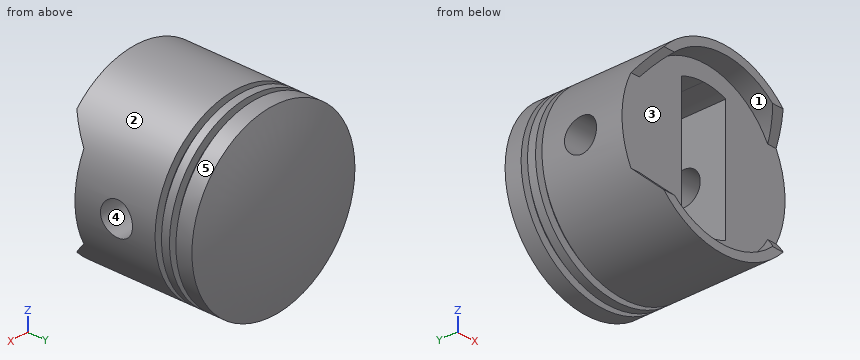
```python
from build123d import *

# Parameters (mm, degrees)
CUT_EXTRUDE_2_DEPTH      = 39.105117767
CUT_EXTRUDE_2_DEPTH_BACK = 39.105117767
SKETCH_4_R               = 4
SKETCH_6_R               = 20
CUT_EXTRUDE_3_DEPTH      = 5
CUT_EXTRUDE_4_DEPTH      = 6
EXTRUDE_1_REACH          = 46.896
EXTRUDE_1_END_RADIUS     = 75


with BuildPart() as part:
    # 草图1 → 旋转3 (revolve)
    with BuildSketch(Plane.XY):
        with BuildLine():
            Line((-22, 9.633147735), (-22, -15.366852265))
            Line((-22, -15.366852265), (0, -15.366852265))
            Line((0, -15.366852265), (0, 22))
            ThreePointArc((0, 22), (-11.113381048, 21.204227615), (-22, 18.833147735))
            Line((-22, 18.833147735), (-22, 14.833147735))
            Line((-22, 14.833147735), (-20, 14.833147735))
            Line((-20, 14.833147735), (-20, 13.233147735))
            Line((-20, 13.233147735), (-22, 13.233147735))
            Line((-22, 13.233147735), (-22, 11.233147735))
            Line((-22, 11.233147735), (-20, 11.233147735))
            Line((-20, 11.233147735), (-20, 9.633147735))
            Line((-20, 9.633147735), (-22, 9.633147735))
        make_face()
    revolve(axis=Axis((0, 22, 0), (0, -1, 0)))

    # 草图4 → 切除-拉伸2 (cut, two sides: drawn at the far end of the back side and taken through both)
    with BuildSketch(Plane(origin=(0, 0, 0), x_dir=(0, 0, -1), z_dir=(1, 0, 0)).offset(-CUT_EXTRUDE_2_DEPTH_BACK)):
        Circle(SKETCH_4_R)
        Polygon((-15, -15.366852265), (-10, -10.366852265), (10, -10.366852265), (15, -15.366852265), align=None)
    extrude(amount=CUT_EXTRUDE_2_DEPTH + CUT_EXTRUDE_2_DEPTH_BACK, mode=Mode.SUBTRACT)

    # 草图6 → 切除-拉伸3 (cut)
    with BuildSketch(Plane.XZ.offset(15.366852265)):
        with Locations(Location((0, 0, 0), (0, 0, 180))):
            Circle(SKETCH_6_R)
    extrude(amount=-CUT_EXTRUDE_3_DEPTH, mode=Mode.SUBTRACT)

    # 草图8 → 切除-拉伸4 (cut, symmetric)
    with BuildSketch(Plane(origin=(0, 0, 0), x_dir=(0, 0, -1), z_dir=(1, 0, 0))):
        with BuildLine():
            Line((-16, 17.273460407), (-16, -10.366852265))
            Line((-16, -10.366852265), (16, -10.366852265))
            Line((16, -10.366852265), (16, 17.273460407))
            ThreePointArc((16, 17.273460407), (0, 19), (-16, 17.273460407))
        make_face()
    extrude(amount=CUT_EXTRUDE_4_DEPTH, both=True, mode=Mode.SUBTRACT)

    # 凸台-拉伸1: up to this cylinder (the profile starts inside it)
    extrude_1_end = Plane(origin=(0, -56, 0), z_dir=(1, 0, 0)) * Cylinder(EXTRUDE_1_END_RADIUS, 253.81433, mode=Mode.PRIVATE)
    # 草图9 → 凸台-拉伸1 (add, up to the surface)
    with BuildSketch(Plane.XZ.offset(10.366852265), mode=Mode.PRIVATE) as extrude_1_sk1:
        with BuildLine():
            Line((6, -16), (6, -14.832396974))
            ThreePointArc((6, -14.832396974), (3.056276215, -15.705386837), (3.1e-08, -16))
            Line((3.1e-08, -16), (6, -16))
        make_face()
    extrude_1_tool1 = extrude(extrude_1_sk1.sketch, amount=-EXTRUDE_1_REACH, mode=Mode.PRIVATE) & extrude_1_end
    add(extrude_1_tool1.solids().sort_by_distance((4.511165, -10.366852, -15.652025))[0])
    # 草图9 → 凸台-拉伸1 (add, up to the surface)
    with BuildSketch(Plane.XZ.offset(10.366852265), mode=Mode.PRIVATE) as extrude_1_sk2:
        with BuildLine():
            Line((-6, -16), (3.1e-08, -16))
            ThreePointArc((3.1e-08, -16), (-3.056276184, -15.705386843), (-6, -14.832396974))
            Line((-6, -14.832396974), (-6, -16))
        make_face()
    extrude_1_tool2 = extrude(extrude_1_sk2.sketch, amount=-EXTRUDE_1_REACH, mode=Mode.PRIVATE) & extrude_1_end
    add(extrude_1_tool2.solids().sort_by_distance((-4.511165, -10.366852, -15.652025))[0])
    # 草图9 → 凸台-拉伸1 (add, up to the surface)
    with BuildSketch(Plane.XZ.offset(10.366852265), mode=Mode.PRIVATE) as extrude_1_sk3:
        with BuildLine():
            ThreePointArc((-6, 14.832396974), (-3.056276199, 15.70538684), (0, 16))
            Line((0, 16), (-6, 16))
            Line((-6, 16), (-6, 14.832396974))
        make_face()
    extrude_1_tool3 = extrude(extrude_1_sk3.sketch, amount=-EXTRUDE_1_REACH, mode=Mode.PRIVATE) & extrude_1_end
    add(extrude_1_tool3.solids().sort_by_distance((-4.511165, -10.366852, 15.652025))[0])
    # 草图9 → 凸台-拉伸1 (add, up to the surface)
    with BuildSketch(Plane.XZ.offset(10.366852265), mode=Mode.PRIVATE) as extrude_1_sk4:
        with BuildLine():
            Line((6, 14.832396974), (6, 16))
            Line((6, 16), (0, 16))
            ThreePointArc((0, 16), (3.056276199, 15.70538684), (6, 14.832396974))
        make_face()
    extrude_1_tool4 = extrude(extrude_1_sk4.sketch, amount=-EXTRUDE_1_REACH, mode=Mode.PRIVATE) & extrude_1_end
    add(extrude_1_tool4.solids().sort_by_distance((4.511165, -10.366852, 15.652025))[0])


solid = part.part
```
Verification items for the finished model (mm, model axes). Face numbers are marked on the shaded views. A direction names the side the tool comes from. Coordinates: 2 decimals unless noted, no trailing zeros. Order: outer loops, then holes, each group sorted by start corner. A loop starts at its lowest first (then second) coordinate and runs counter-clockwise, first axis right, second up. Notation, with made-up numbers: (-26, -25.5) -> (-20, -25.5) arc R30 ccw to (-20, 8.5) -> close; hole circle Ø1 at (85.25, 69). An arc over 180 degrees is marked (long way). Put each result on its own line as item: value. Start each with the question number.
1) Cross-section at B-B (z = 0). State how many separate pieces and enclosed holes the cut face has, plus the area to 3 significant figures.
2) Tool access check on the marked faces 1 and 2. Record the directions out of +Z, -Z, +X, -X, +Y, -Y that give a thin tool (end or side, any length) a straight path to the whole face; none if there is none.
3) Cross-section at C-C (x = 15). Enter the section's corners in (y, z).
4) Go/stop test with flat-tipped pins: pin 1 (6.5 mm diameter, centred on y = 0, z = 0, fed in from +X); pin 2 (9 mm diameter, centred on y = 2, z = -5.5, fed in from -X); pin 3 (3 mm diameter, centred on x = -15, y = 2, fed in from +Z); pin 4 (22 mm diameter, centred on x = 1, z = 2, fed in from -Y). Record where each tip stops, or that it passes through.
5) Cross-section at A-A (y = 16). Enter the section's corners in (x, z).
6) Material ranges on L1, parallel to Y at x = 17.5, z = -8; L2, parallel to X at y = 3.5, z = 11; L3, parallel to Z at x = 11.5, y = 0 (3 decimals), recorded low to high.
7) Cross-section at D-D (y = 0). Enter the section's corners in (x, z), plus the area to 3 significant figures.
8) Release check for a two-part mould opening along X. For the marked faces 3, 4 and 5 record: pulls with the +X half, pulls with the -X half, needs draft (parallel to the pull), parting line crosses it, or undercut.
Geometry check:
1. separate pieces: 3
1. enclosed holes: 0
1. area: 757 mm^2
2. face 1: -Y
2. face 2: +Y, -Y
3. outline: (-15.37, -16.09) -> (9.63, -16.09) -> (9.63, -13.23) -> (11.23, -13.23) -> (11.23, -16.09) -> (13.23, -16.09) -> (13.23, -13.23) -> (14.83, -13.23) -> (14.83, -16.09) -> (18.83, -16.09) arc R76.54 ccw to (18.83, 16.09) -> (14.83, 16.09) -> (14.83, 13.23) -> (13.23, 13.23) -> (13.23, 16.09) -> (11.23, 16.09) -> (11.23, 13.23) -> (9.63, 13.23) -> (9.63, 16.09) -> (-15.37, 16.09) -> (-15.37, 15) -> (-13.6, 13.23) -> (-10.37, 13.23) -> (-10.37, -13.23) -> (-13.6, -13.23) -> (-15.37, -15) -> close; hole circle Ø8 at (0, 0)
4. pin 1: passes through
4. pin 2: stops at x = -21.96
4. pin 3: stops at z = 17.37
4. pin 4: stops at y = -10.37
5. outline: circle Ø44 at (0, 0); hole (-6, -14.83) arc R16 ccw to (6, -14.83) -> (6, 14.83) arc R16 ccw to (-6, 14.83) -> close
6. L1: y = -10.37 to 19.59
6. L2: x = -19.05 to -6, 6 to 19.05
6. L3: z = -18.755 to -4, 4 to 18.755
7. outline: (-21.63, -4) arc R22 ccw to (21.63, -4) -> (6, -4) -> (6, -14.83) arc R16 cw to (-6, -14.83) -> (-6, -4) -> close; (-21.63, 4) -> (-6, 4) -> (-6, 14.83) arc R16 cw to (6, 14.83) -> (6, 4) -> (21.63, 4) arc R22 ccw to start
7. area: 892 mm^2
8. face 3: undercut
8. face 4: needs draft
8. face 5: parting line crosses it
